```python
from build123d import *

# Parameters (mm, degrees)
BOSS_EXTRUDE1_DEPTH = 140
FILLET1_R           = 10


with BuildPart() as part:
    # Sketch1 → Boss-Extrude1 (new body)
    with BuildSketch(Plane(origin=(0, 0, 0), x_dir=(0, 0, -1), z_dir=(1, 0, 0))):
        with BuildLine():
            ThreePointArc((4, 50), (0.381966011, 52.236067977), (0, 48))
            Line((0, 48), (0, 50))
            Line((0, 50), (3, 50))
            Line((3, 50), (3, 48))
            ThreePointArc((3, 48), (3.736067977, 48.881966011), (4, 50))
        make_face()
        with BuildLine():
            Line((0, 50), (0, 48))
            ThreePointArc((0, 48), (1.5, 47.5), (3, 48))
            Line((3, 48), (3, 50))
            Line((3, 50), (0, 50))
        make_face()
        with BuildLine():
            Line((0, 48), (0, 0))
            Line((0, 0), (3, 0))
            Line((3, 0), (3, 48))
            ThreePointArc((3, 48), (1.5, 47.5), (0, 48))
        make_face()
    extrude(amount=BOSS_EXTRUDE1_DEPTH)

    # Fillet1
    # the kernel refuses this fillet: 10 mm, written as the material it takes off along each edge
    with BuildSketch(Plane(origin=(-17.853571071, 0, 0), x_dir=(0, 1, 0), z_dir=(1, 0, 0))) as fillet1_piece_1:
        with BuildLine():
            CenterArc((7.141428429, -10), FILLET1_R, 90, 45.572995999)
            Line((0, -3), (-0.142828569, -2.86))
            ThreePointArc((-0.142828569, -2.86), (-0.2, -1.5), (-0.2, 0))
            Line((-0.2, 0), (0, 0.2))
            Line((0, 0.2), (7.141428429, 0.2))
            Line((7.141428429, 0.2), (7.141428429, 0))
        make_face()
    extrude(amount=175.707142143, mode=Mode.SUBTRACT)


solid = part.part
```
For this review, take the finished solid that the model builds, in its own axes (mm). A direction names the side the tool comes from. Give positions to 0.01 mm unless a question says otherwise; leave off trailing zeros. Order: outer loops, then holes, each group sorted by start corner. A loop starts at its lowest first (then second) coordinate and runs counter-clockwise, first axis right, second up.
1) Wall thickness on line 1 (Z direction, x = 92.5, y = 31); line 2 (Y direction, x = 19.5, z = -1.5); line 3 (Y direction, x = 67.5, z = -1): over which ranges is each line inside the solid? List them lowest first.
2) Insertion check: pin 1 (1.5 mm diameter, centred on x = 52.5, z = -0.5, fed in from +Y); pin 2 (3 mm diameter, centred on x = 111.5, y = 23.5, fed in from +Z); pin 3 (1.5 mm diameter, centred on y = 29, z = -1.5, fed in from -X); pin 4 (1.5 mm diameter, centred on x = 88, z = -0.5, fed in from -Y). Each pin has a flat end and moves straight along its axis. Give the tip position at first contact, or say it passes through.
3) Take a section at B-B (z = -1.45). Give the boundary of the cut face in (x, y).
4) For faces 1 (the face through (140, 27, -1)), 2 (the face through (69, 24, -3)), 3 (the face through (69, 28, 0)), list the 3-axis set-ups (+Z, -Z, +X, -X, +Y, -Y) from which the entire face can be reached by the end or side of a thin tool; tool diameter is ignored.
5) Take a section at A-A (x = 33). Give the boundary of the cut face in (y, z).
6) Take a section at C-C (y = 24). Give the boundary of the cut face in (x, z), then the cut area to 3 significant figures.
Derived:
1. line 1: z = -3 to 0
1. line 2: y = 1.87 to 52.5
1. line 3: y = 2.78 to 52.45
2. pin 1: stops at y = 52.49
2. pin 2: stops at z = 0
2. pin 3: stops at x = 0
2. pin 4: stops at y = 2.3
3. outline: (0, 1.96) - (140, 1.96) - (140, 52.5) - (0, 52.5) - close
4. face 1: +Z, -Z, +X, +Y, -Y
4. face 2: -Z, +X, -X, -Y
4. face 3: +Z, +X, -X, -Y
5. outline: (0, -3) - (48, -3) arc R2.5 ccw (long way) to (48, 0) - (7.14, 0) arc R10 ccw to start
6. outline: (0, -3) - (140, -3) - (140, 0) - (0, 0) - close
6. area: 420 mm2
